Here's the drawing with two shaded views (mm, measured from the low corner). I have some questions. A direction names the side the tool comes from. Round coordinates to 2 decimals unless told otherwise and drop trailing zeros. Order: outer loops, then holes, each group sorted by start corner. A loop starts at its lowest first (then second) coordinate and runs counter-clockwise, first axis right, second up.
Q1. Will this pin go through, and if not, where does the flat tip stop? P1, Ø4, axis at y = 6, z = 14.5, coming from the +X side.
Q2. If we section it at A-A (x = 7.25): Please give me the cut outline in (y, z) (1 decimal).
Q3. For the marked faces 4 and 5, which set-ups out of +Z, -Z, +X, -X, +Y, -Y let a thin tool reach every point of the face, with its end or its side?
Q4. We'd pull the mould along X, two halves only. Please class the marked faces 1, 2 and 3: pulls with the +X half, pulls with the -X half, needs draft (parallel to the pull), parting line crosses it, or undercut.
Q5. If we section it at B-B (z = 5.5): Please give me the cut outline in (x, y) (1 decimal).
Q6. If I drill on line 1 (Z direction, x = 7, y = 5.75) (1 decimal); line 2 (Z direction, x = 6.5, y = 6.5) (1 decimal); line 3 (X direction, y = 3, z = 6.25) (1 decimal), over which ranges is the centre line in solid material (lowest first)?
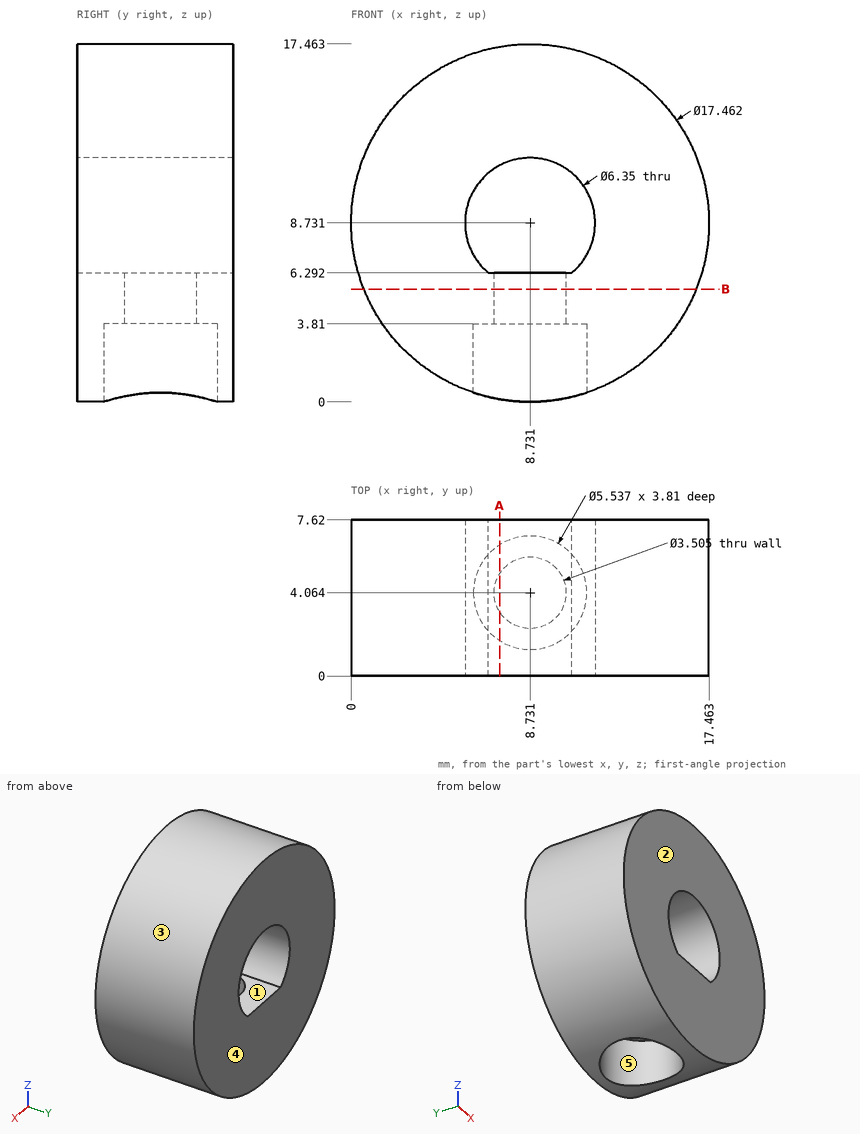
Solution:
1. P1: stops at x = 16.61
2. outline: (0, 0.1) - (1.7, 0.1) - (1.7, 3.8) - (3.1, 3.8) - (3.1, 6.3) - (0, 6.3) - close; (0, 11.5) - (7.6, 11.5) - (7.6, 17.3) - (0, 17.3) - close; (5, 3.8) - (6.4, 3.8) - (6.4, 0.1) - (7.6, 0.1) - (7.6, 6.3) - (5, 6.3) - close
3. face 4: +Z, -Z, +X, -X, +Y
3. face 5: -Z
4. face 1: undercut
4. face 2: needs draft
4. face 3: parting line crosses it
5. outline: (0.6, 0) - (16.8, 0) - (16.8, 7.6) - (0.6, 7.6) - close; hole circle Ø3.5 at (8.7, 4.1)
6. line 1: z = 3.8 to 6.3, 11.4 to 17.3
6. line 2: z = 0.3 to 6.5, 11 to 17.2
6. line 3: x = 0.4 to 7.3, 10.1 to 17.1
